Here's how the part is built. I have some questions about the finished solid (model axes, mm). Face numbers are marked on the shaded views. A direction names the side the tool comes from. Give positions to 0.01 mm unless a question says otherwise; leave off trailing zeros. Loops run counter-clockwise (first coordinate to the right, second up) from the corner with the lowest first, then second, coordinate; pieces in that order, holes last.
Q1. For the marked faces 5 and 6, which set-ups out of +Z, -Z, +X, -X, +Y, -Y let a thin tool reach every point of the face, with its end or its side?
Q2. Thinking about a two-plate mould opening in X: for the marked faces 1, 2, 3 and 4, which applies, pulls with the +X half, pulls with the -X half, needs draft (parallel to the pull), parting line crosses it, or undercut?
Q3. Suppose I cut it at D-D (z = 7.5). List the corners of the cut face in (x, y) for me.
Q4. I need wall thicknesses on probe 1 along X at (y, z) = (0, -7.8); probe 2 along Z at (x, y) = (-6.5, 1.25). Which ranges of each line are inside material? Lowest first, please.
Q5. I'm going to push flat-ended pins straight in: P1, Ø1.5, axis at x = 0, z = 0.5, coming from the +Y side; P2, Ø5, axis at y = 5, z = 10, coming from the +X side; P3, Ø1, axis at y = -3, z = 12.5, coming from the +X side; P4, Ø3, axis at x = 1, y = -0.5, coming from the -Z side. Where does each tip first touch, or does it pass through?
Q6. Suppose I cut it at C-C (z = 20.5). List the corners of the cut face in (x, y) for me.
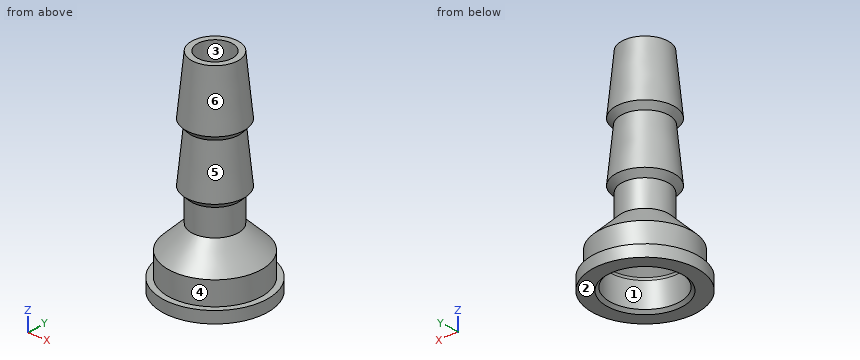
```python
from build123d import *

# Parameters (mm, degrees)
F2_R        = 3
F3_DEPTH    = 35.5362252722
F4_T4_ANGLE = 180
F4_T6_ANGLE = 180


# Not quite as in the source:
# - a fillet or chamfer that OpenCascade refuses, or shapes differently, is made with other operations: its cross-section is extruded or revolved along the edge and cut away or added
# - a feature names something its author has since deleted; it is built from what else it names


with BuildPart() as f1:
    # F0 (on Front) → F1 (revolve)
    with BuildSketch(Plane.XZ):
        Polygon((-6, -5.5352252722), (0, 0.4647747278), (0, 25), (-4, 25), (-5, 15), (-4.099503719, 14.0049628098), (-5, 5), (-4, 4), (-4, -0.5352252722), (-8, -4.5352252722), (-8, -8.5352252722), (-9, -8.5352252722), (-9, -10.5352252722), (-6, -10.5352252722), align=None)
    revolve(axis=Axis((0, 0, 12.7323873639), (0, 0, 1)))

    # F2 (on face) → F3 (cut, through all)
    with BuildSketch(Plane.XY.offset(25)):
        Circle(F2_R)
    extrude(amount=-F3_DEPTH, mode=Mode.SUBTRACT)

    # F4: chamfer of 0.5 on 4 edges, made by hand

    # F4_s1 → F4_t2 (revolve)
    with BuildSketch(Plane.XZ):
        Polygon((-5.8535533906, -5.3887786628), (-6, -5.7423320534), (-6, -5.5352252722), align=None)
    revolve(axis=Axis((0, 0, -5.5352252722), (0, 0, 1)))

    # F4_s3 → F4_t4 (revolve, cut)
    with BuildSketch(Plane.XZ):
        Polygon((-3.1464466094, -2.6816718816), (-3, -2.328118491), (-3, -2.5352252722), align=None)
    revolve(axis=Axis((0, 0, -2.5352252722), (0, 0, 1)), revolution_arc=F4_T4_ANGLE, mode=Mode.SUBTRACT)

    # F4_s5 → F4_t6 (revolve, cut)
    with BuildSketch(Plane.XZ):
        Polygon((3.1464466094, -2.6816718816), (3, -2.328118491), (3, -2.5352252722), align=None)
    revolve(axis=Axis((0, 0, -2.5352252722), (0, 0, 1)), revolution_arc=F4_T6_ANGLE, mode=Mode.SUBTRACT)

    # F4_s7 → F4_t8 (revolve, cut)
    with BuildSketch(Plane.XZ):
        Polygon((-6, -10.0352252722), (-6.5, -10.5352252722), (-6, -10.5352252722), align=None)
    revolve(axis=Axis((0, 0, -10.5352252722), (0, 0, 1)), mode=Mode.SUBTRACT)


solid = f1.part
```
Solutions:
1. face 5: none
1. face 6: +Z
2. face 1: undercut
2. face 2: needs draft
2. face 3: undercut
2. face 4: parting line crosses it
3. outline: circle Ø9.5 at (0, 0); hole circle Ø6 at (0, 0)
4. probe 1: x = -8 to -6, 6 to 8
4. probe 2: z = -10.54 to -3.15
5. P1: stops at y = 4
5. P2: stops at x = 3.77
5. P3: stops at x = 3.44
5. P4: passes through
6. outline: circle Ø8.9 at (0, 0); hole circle Ø6 at (0, 0)
